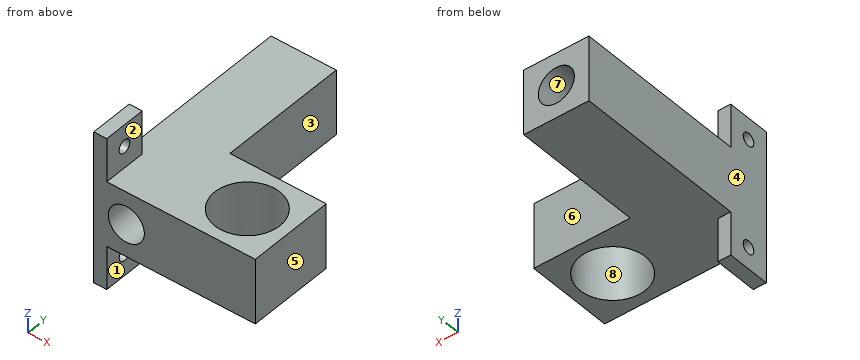
from build123d import *

# Parameters (mm, degrees)
SKETCH1_R           = 7.5
BOSS_EXTRUDE1_DEPTH = 15
SKETCH2_R           = 4.15
CUT_EXTRUDE1_DEPTH  = 59.853707622
SKETCH3_W           = 35
SKETCH3_H           = 10
SKETCH3_R           = 1.5
BOSS_EXTRUDE2_DEPTH = 3


with BuildPart() as part:
    # Sketch1 → Boss-Extrude1 (new body)
    with BuildSketch(Plane.XY):
        Polygon((-12.180119589, 10), (-12.180119589, 40), (-27.180119589, 40), (-27.180119589, -10), (10, -10), (10, 10), align=None)
        Circle(SKETCH1_R, mode=Mode.SUBTRACT)
    extrude(amount=BOSS_EXTRUDE1_DEPTH)

    # Sketch2 → Cut-Extrude1 (cut, through all)
    with BuildSketch(Plane(origin=(0, 40, 0), x_dir=(1, 0, 0), z_dir=(0, 1, 0))):
        with Locations(Location((-19.680119589, -7.5, 0), (0, 0, 270))):
            Circle(SKETCH2_R)
    extrude(amount=-CUT_EXTRUDE1_DEPTH, mode=Mode.SUBTRACT)

    # Sketch3 → Boss-Extrude2 (add)
    with BuildSketch(Plane.ZY.offset(27.180119589)):
        with Locations((7.5, -5)):
            Rectangle(SKETCH3_W, SKETCH3_H)
        with Locations((-5, -5)):
            Circle(SKETCH3_R, mode=Mode.SUBTRACT)
        with Locations((20, -5)):
            Circle(SKETCH3_R, mode=Mode.SUBTRACT)
    extrude(amount=-BOSS_EXTRUDE2_DEPTH)


solid = part.part
CAD build for the part. Positions are in the model's coordinates, mm. Face numbers are marked on the shaded views. A direction names the side the tool comes from. Round coordinates to 2 decimals unless told otherwise and drop trailing zeros. Loops run counter-clockwise (first coordinate to the right, second up) from the corner with the lowest first, then second, coordinate; pieces in that order, holes last. Notation, with made-up numbers: (34, 75) - (52, 75) arc R19 cw to (52, 103) - close; hole circle Ø7 at (-7.5, 53). An arc over 180 degrees is marked (long way). Put each result on its own line as item: value.
1. Wall check: line 1 (X direction, y = 35.5, z = 7.5); line 2 (X direction, y = -6, z = 8); line 3 (Y direction, x = 0, z = 5.5). Give the ranges that are in metal, low to high.
Geometry check:
line 1: -27.18 to -23.83, -15.53 to -12.18
line 2: -27.18 to -23.8, -15.56 to -4.5, 4.5 to 10
line 3: -10 to -7.5, 7.5 to 10
2. Slice it at B-B on y = -5. List the corners of the cut face in (x, z).
Geometry check:
outline: (-27.18, -10) - (-24.18, -10) - (-24.18, -6.5) - (-27.18, -6.5) - close; (-27.18, -3.5) - (-24.18, -3.5) - (-24.18, 0) - (-5.59, 0) - (-5.59, 15) - (-24.18, 15) - (-24.18, 18.5) - (-27.18, 18.5) - close; (-27.18, 21.5) - (-24.18, 21.5) - (-24.18, 25) - (-27.18, 25) - close; (5.59, 0) - (10, 0) - (10, 15) - (5.59, 15) - close; hole circle Ø8.3 at (-19.68, 7.5)
3. Two-plate mould, pull along X, no slides. Class the marked faces 5, 6, 7 and 8: released by +X, released by -X, zero draft, split by the parting line, or undercut.
Geometry check:
face 5: released by +X
face 6: zero draft
face 7: undercut
face 8: undercut
4. Slice it at D-D on z = 20. List the corners of the cut face in (x, y), and give its area (3 significant figures).
Geometry check:
outline: (-27.18, -10) - (-24.18, -10) - (-24.18, -6.5) - (-27.18, -6.5) - close; (-27.18, -3.5) - (-24.18, -3.5) - (-24.18, 0) - (-27.18, 0) - close
area: 21.0 mm²
5. 3-axis set-ups, long thin cutter, end or side, ignore diameter. For the marked faces 1, 2, 3 and 4: which of +Z, -Z, +X, -X, +Y, -Y reach the whole face in a straight line?
Geometry check:
face 1: -Z, +X, +Y, -Y
face 2: +Z, +X, +Y, -Y
face 3: +Z, -Z, +X, +Y
face 4: +Z, -Z, -X, +Y, -Y
6. Slice it at A-A on z = 7.5. List the corners of the cut face in (x, y).
Geometry check:
outline: (-27.18, -10) - (-23.83, -10) - (-23.83, 40) - (-27.18, 40) - close; (-15.53, -10) - (10, -10) - (10, 10) - (-12.18, 10) - (-12.18, 40) - (-15.53, 40) - close; hole circle Ø15 at (0, 0)
7. Slice it at C-C on x = 0. List the corners of the cut face in (y, z), and give its area (3 significant figures).
Geometry check:
outline: (-10, 0) - (-7.5, 0) - (-7.5, 15) - (-10, 15) - close; (7.5, 0) - (10, 0) - (10, 15) - (7.5, 15) - close
area: 75.0 mm²
8. Pin check, flat tips, straight feed: P1, Ø17, axis at x = 0, y = 0, coming from the -Z side; P2, Ø8, axis at y = -4, z = -6.5, coming from the +X side; P3, Ø1, axis at y = 33.5, z = 9, coming from the +X side. Stop position of each tip, or through.
Geometry check:
P1: z = 0
P2: x = -24.18
P3: x = -12.18
